CAD build for the part. Positions are in the model's coordinates, mm. A direction names the side the tool comes from. Round coordinates to 2 decimals unless told otherwise and drop trailing zeros. Loops run counter-clockwise (first coordinate to the right, second up) from the corner with the lowest first, then second, coordinate; pieces in that order, holes last. Notation, with made-up numbers: (88.25, 23.5) -> (103.25, 23.5) arc R22 ccw to (103.25, 59.5) -> close; hole circle Ø1 at (9.5, 2.25). An arc over 180 degrees is marked (long way). Answer as CSV lines item,"result".
Autodesk Inventor part; units mm, degrees
ref_plane "YZ Plane" through (0, 0, 0) normal (1, 0, 0) x (0, 1, 0)
ref_plane "XZ Plane" through (0, 0, 0) normal (0, 1, 0) x (-1, 0, 0)
ref_plane "XY Plane" through (0, 0, 0) normal (0, 0, 1) x (1, 0, 0)
sketch "Sketch1" plane through (0, 0, 0) normal (1, 0, 0) x (0, 1, 0)
  line L0 (0, 0) -> (50.8, 0)
  line L1 (0, 133.35) -> (0, 184.15)
  line L2 (0, 184.15) -> (73.025, 184.15)
  line L3 (73.025, 184.15) -> (73.025, 133.35)
  line L4 (69.85, 180.975) -> (3.175, 180.975)
  line L5 (3.175, 180.975) -> (3.175, 136.525)
  line L6 (69.85, 136.525) -> (69.85, 180.975)
  line L7 (29.2989, 148.3694) -> (29.2989, 120.4477)
  line L8 (41.9989, 148.9666) -> (41.9989, 122.6874)
  line L9 (0, 133.35) -> (29.2989, 133.35)
  line L10 (41.9989, 133.35) -> (73.025, 133.35)
  line L11 (3.175, 136.525) -> (29.2989, 136.525)
  line L12 (41.9989, 136.525) -> (69.85, 136.525)
  point P0 (3.175, 180.975)
  point P1 (69.85, 136.525)
  dimension "d0" = 50.8
  dimension "d3" = 50.8
  dimension "d4" = 73.025
  dimension "d5" = 3.175
  dimension "d6" = 3.175
  dimension "d7" = 3.175
  dimension "d8" = 3.175
  dimension "d9" = 3.175
  dimension "d11" = 3.175
  dimension "d13" = 26.1239
  dimension "d14" = 12.7
  dimension "d16" = 133.35
  dimension "d17" = 3.175
  dimension "d18" = 3.175
revolve "Revolution1" add sketch "Sketch1" angle 180 about axis through (0, 0, 0) along (0, 1, 0)
sketch "Sketch2" plane through (0, 73.025, 184.15) normal (0, 1, 0) x (1, 0, 0)
  point P0 (0, 184.15)
properties part number "Outer_Shell"
Q1. Slice it at A-A, the plane y = 53. Give the cut face in (x, z) (3 decimals).
Results:
outline,"(0, -184.15) arc R184.15 ccw to (0, 184.15) -> (0, 180.975) arc R180.975 cw to (0, -180.975) -> close; (0, -136.525) arc R136.525 ccw to (0, 136.525) -> (0, 133.35) arc R133.35 cw to (0, -133.35) -> close"
Q2. Slice it at D-D, the plane x = 121.5. Give the cut face in (y, z) (3 decimals).
Results:
outline,"(0, -138.38) -> (73.025, -138.38) -> (73.025, -54.954) -> (41.999, -54.954) -> (41.999, -62.264) -> (69.85, -62.264) -> (69.85, -134.126) -> (3.175, -134.126) -> (3.175, -62.264) -> (29.299, -62.264) -> (29.299, -54.954) -> (0, -54.954) -> close; (0, 54.954) -> (29.299, 54.954) -> (29.299, 62.264) -> (3.175, 62.264) -> (3.175, 134.126) -> (69.85, 134.126) -> (69.85, 62.264) -> (41.999, 62.264) -> (41.999, 54.954) -> (73.025, 54.954) -> (73.025, 138.38) -> (0, 138.38) -> close"
Q3. Slice it at C-C, the plane z = 0. Give the cut face in (x, y) (3 decimals), and give its area (3 significant figures).
Results:
outline,"(133.35, 0) -> (184.15, 0) -> (184.15, 73.025) -> (133.35, 73.025) -> (133.35, 41.999) -> (136.525, 41.999) -> (136.525, 69.85) -> (180.975, 69.85) -> (180.975, 3.175) -> (136.525, 3.175) -> (136.525, 29.299) -> (133.35, 29.299) -> close"
area,"706 mm2"
Q4. Drop flat-ended pins along their axis: pin 1 Ø8 at (y, z) = (25.5, 115.5) entering from -X; pin 2 Ø10 at (x, y) = (37, 11.5) entering from +Z; pin 3 Ø3 at (x, y) = (79.5, 42.5) entering from +Z. Give the stop position or say it passes through.
Results:
pin 1,"x = 59.18"
pin 2,"z = 181.35"
pin 3,"z = 166.81"
Q5. Probe L1, parallel to Y at x = 41.5, z = 162 (3 decimals); L2, parallel to Z at x = 124, y = 4.5; L3, parallel to Z at x = 23, y = 7. List the from-to ranges inside material, lowest first. Write a range as [from, to].
Results:
L1,"[0, 3.175], [69.85, 73.025]"
L2,"[-136.14, -131.82], [-57.12, -49.05], [49.05, 57.12], [131.82, 136.14]"
L3,"[-182.71, -179.51], [-134.57, -131.35], [131.35, 134.57], [179.51, 182.71]"
Q6. Tool access for faces 4 (the cylindrical face through (184.105, 37.024, 4.049)), 5 (the cylindrical face through (180.93, 36.05, -3.98)), 6 (the flat face through (134, 41.999, -1)): list every direction of +Z, -Z, +X, -X, +Y, -Y with a clear straight run to the whole face (end or side of a thin tool).
Results:
face 4,"+X, +Y, -Y"
face 5,"none"
face 6,"-X"
Q7. Two-plate mould, pull along Y, no slides. Class faces 1 (the flat face through (138, 69.85, -14)), 2 (the flat face through (134, 73.025, -3)), 3 (the flat face through (0, 33.6, -181.4)): pulls with the +Y half, pulls with the -Y half, needs draft (parallel to the pull), parting line crosses it, or undercut.
Results:
face 1,"undercut"
face 2,"pulls with the +Y half"
face 3,"needs draft"
Q8. Slice it at B-B, the plane x = 168. Give the cut face in (y, z) (3 decimals), and give its area (3 significant figures).
Results:
outline,"(0, -75.414) -> (73.025, -75.414) -> (73.025, 75.414) -> (0, 75.414) -> close; hole (3.175, -67.29) -> (69.85, -67.29) -> (69.85, 67.29) -> (3.175, 67.29) -> close"
area,"2,040 mm2"
